from build123d import *

# Parameters (mm, degrees)
F1_DEPTH = 3
F3_DEPTH = 3
F5_DEPTH = 3
F7_DEPTH = 3
F8_R     = 15
F9_DEPTH = 3


with BuildPart() as f1:
    # F0 (on Top) → F1 (new body)
    with BuildSketch(Plane.XY):
        Polygon((16.18034, 63.244295), (0, 75), (-16.18034, 63.244295), (-13.241414, 59.19921), (-15.506661, 57.553411), (-18.445587, 61.598496), (-52.883651, 36.577778), (-49.944725, 32.532693), (-52.209973, 30.886895), (-55.148899, 34.93198), (-71.329239, 23.176275), (-65.148899, 4.155144), (-60.393616, 5.700229), (-59.528369, 3.037271), (-64.283651, 1.492186), (-51.129481, -38.992186), (-46.374199, -37.447101), (-45.508951, -40.110059), (-50.264234, -41.655144), (-44.083894, -60.676275), (-24.083894, -60.676275), (-24.083894, -55.676275), (-21.283894, -55.676275), (-21.283894, -60.676275), (21.283894, -60.676275), (21.283894, -55.676275), (24.083894, -55.676275), (24.083894, -60.676275), (44.083894, -60.676275), (50.264234, -41.655144), (45.508951, -40.110059), (46.374199, -37.447101), (51.129481, -38.992186), (64.283651, 1.492186), (59.528369, 3.037271), (60.393616, 5.700229), (65.148899, 4.155144), (71.329239, 23.176275), (55.148899, 34.93198), (52.209973, 30.886895), (49.944725, 32.532693), (52.883651, 36.577778), (18.445587, 61.598496), (15.506661, 57.553411), (13.241414, 59.19921), align=None)
        Polygon((-57.063391, 18.54102), (0, 60), (57.063391, 18.54102), (35.267115, -48.54102), (-35.267115, -48.54102), align=None, mode=Mode.SUBTRACT)
    extrude(amount=F1_DEPTH)

    # F2 (on face) → F3 (join)
    with BuildSketch(Plane.XY.offset(3)):
        Polygon((-57.063391, -18.54102), (0, -60), (57.063391, -18.54102), (35.267115, 48.54102), (-35.267115, 48.54102), align=None)
        Polygon((47.552826, -15.45085), (0, -50), (-47.552826, -15.45085), (-29.389263, 40.45085), (29.389263, 40.45085), align=None, mode=Mode.SUBTRACT)
    extrude(amount=-F3_DEPTH)

    # F4 (on face) → F5 (join)
    with BuildSketch(Plane.XY.offset(3)):
        Polygon((42.797543, 13.905765), (0, 45), (-42.797543, 13.905765), (-26.450336, -36.405765), (26.450336, -36.405765), align=None)
        Polygon((-33.286978, 10.815595), (0, 35), (33.286978, 10.815595), (20.572484, -28.315595), (-20.572484, -28.315595), align=None, mode=Mode.SUBTRACT)
    extrude(amount=-F5_DEPTH)

    # F6 (on face) → F7 (join)
    with BuildSketch(Plane.XY.offset(3)):
        Polygon((-33.286978, -10.815595), (0, -35), (33.286978, -10.815595), (20.572484, 28.315595), (-20.572484, 28.315595), align=None)
        Polygon((23.776413, -7.725425), (0, -25), (-23.776413, -7.725425), (-14.694631, 20.225425), (14.694631, 20.225425), align=None, mode=Mode.SUBTRACT)
    extrude(amount=-F7_DEPTH)

    # F8 (on face) → F9 (join)
    with BuildSketch(Plane.XY.offset(3)):
        Polygon((-14.530851, -20), (14.530851, -20), (23.51141, 7.63932), (0, 24.72136), (-23.51141, 7.63932), align=None)
        Circle(F8_R, mode=Mode.SUBTRACT)
    extrude(amount=-F9_DEPTH)


solid = f1.part
Geometry: final body of the model. Coordinates: model frame, mm. A direction names the side the tool comes from. Give positions to 0.01 mm unless a question says otherwise; leave off trailing zeros. Write each loop counter-clockwise with the first axis right and the second up, starting at its lowest first coordinate (ties: lowest second). Pieces come first, ordered by that corner, then holes. Notation, with made-up numbers: M 48.5,-11.5 L 104.5,-11.5 A12 ccw 104.5,6.5 Z; hole C 6,57.5 d10. An arc over 180 degrees is marked long. Answer in a Markdown table with one row per item. Add a question column.
(1) Mould query, pull axis Y, two halves, no side actions, for faces 1 (the flat face through (-7.98, 69.2, 1.48)), 2 (the flat face through (-16.75, -22.83, 1.52)), 3 (the flat face through (-34, -60.676, 1)). Classes: +Y half, -Y half, draft (parallel to the pull), parting line (faces both ways), or undercut.
(2) Section A-A on y = -45. Return loops of the section in (x, z), and give its area (3 significant figures).
(3) First-contact query: pin 1 (1.5 mm diameter, centred on x = 4.5, z = 1.5, fed in from +Y); pin 2 (0.9 mm diameter, centred on x = 1, z = 1, fed in from +Y); pin 3 (18 mm diameter, centred on x = 0, y = 0, fed in from -Z); pin 4 (0.9 mm diameter, centred on y = -57, z = 2, fed in from -X). Flat tips, straight axial feed; report the tip coordinate or a pass-through.
(4) Section C-C on z = 1.4. State how many separate pieces and enclosed holes the cut face has, and give its area (3 significant figures).
(5) Section B-B on x = -11.5. Return loops of the section in (y, z), and give its area (3 significant figures).
(6) Reachability of faces 4 (the flat face through (21.284, -58, 1)), 5 (the flat face through (47.92, -40.893, 1.479)), 6 (the flat face through (-35.424, 49.263, 1.479)), 7 (the flat face through (43.551, -3.135, 1.521)) from +Z, -Z, +X, -X, +Y, -Y: full face, straight path, thin tool, end or side. Return the list, or none.
(7) Ray query, line 1 (Y direction, x = 0, z = 0.7); line 2 (X direction, y = -15.5, z = 2.4); line 3 (X direction, y = -21.5, z = 1.3). Return the intervals inside material, ascending.
Result set:
| question | item | result |
|---|---|---|
| 1 | face 1 | +Y half |
| 1 | face 2 | undercut |
| 1 | face 3 | -Y half |
| 2 | outline | M -49.18,0 L -36.42,0 L -36.42,3 L -49.18,3 Z; M -20.65,0 L -6.88,0 L -6.88,3 L -20.65,3 Z; M 6.88,0 L 20.65,0 L 20.65,3 L 6.88,3 Z; M 36.42,0 L 49.18,0 L 49.18,3 L 36.42,3 Z |
| 2 | area | 159 mm^2 |
| 3 | pin 1 | stops at y = 72.28 |
| 3 | pin 2 | stops at y = 74.6 |
| 3 | pin 3 | passes through |
| 3 | pin 4 | stops at x = -45.42 |
| 4 | separate pieces | 1 |
| 4 | enclosed holes | 21 |
| 4 | area | 9,890 mm^2 |
| 5 | outline | M -60.68,0 L -41.64,0 L -41.64,3 L -60.68,3 Z; M -36.41,0 L -28.32,0 L -28.32,3 L -36.41,3 Z; M -26.64,0 L -9.63,0 L -9.63,3 L -26.64,3 Z; M 9.63,0 L 16.37,0 L 16.37,3 L 9.63,3 Z; M 20.23,0 L 36.64,0 L 36.64,3 L 20.23,3 Z; M 40.45,0 L 48.54,0 L 48.54,3 L 40.45,3 Z; M 51.64,0 L 66.64,0 L 66.64,3 L 51.64,3 Z |
| 5 | area | 271 mm^2 |
| 6 | face 4 | +Z, -Z, -Y |
| 6 | face 5 | +Z, -Z, +X |
| 6 | face 6 | +Z, -Z, -X, +Y |
| 6 | face 7 | +Z, -Z |
| 7 | line 1 | y = -60.68 to -48.54, -36.41 to -25, -20 to -15, 15 to 28.32, 35 to 48.54, 60 to 75 |
| 7 | line 2 | x = -58.76 to -46, -33.24 to 33.24, 46 to 58.76 |
| 7 | line 3 | x = -56.81 to -39.23, -31.29 to -22.79, -18.58 to -4.82, 4.82 to 18.58, 22.79 to 31.29, 39.23 to 56.81 |
